from build123d import *
from OCP.BRepAlgoAPI import BRepAlgoAPI_Cut
from OCP.TopTools import TopTools_ListOfShape

# Parameters (mm, degrees)
BOSS_EXTRUDE1_START = -68.064063
BOSS_EXTRUDE1_DEPTH = 898.128125
CUT_EXTRUDE1_START  = -21.828125
SKETCH2_R           = 10.589945851
SKETCH2_R_2         = 7.9375
CUT_EXTRUDE1_DEPTH  = 21.828125
CUT_EXTRUDE2_START  = -898.128125
SKETCH2_2_R         = 10.589945851
SKETCH2_2_R_2       = 7.9375
CUT_EXTRUDE2_DEPTH  = 21.828125


with BuildPart() as part:
    # Sketch1 → Boss-Extrude1 (new body)
    with BuildSketch(Plane.XY.offset(BOSS_EXTRUDE1_START)):
        with BuildLine():
            Line((4.035093565, -9.791065981), (3.586322342, -7.081115612))
            ThreePointArc((3.586322342, -7.081115612), (-1.296798787, 7.830850475), (-1.112187943, -7.859194884))
            Line((-1.112187943, -7.859194884), (-0.663416719, -10.569145253))
            Line((-0.663416719, -10.569145253), (4.035093565, -9.791065981))
        make_face()
    extrude(amount=BOSS_EXTRUDE1_DEPTH)

    # Sketch2 → Cut-Extrude1 (cut)
    with BuildSketch(Plane.XY.offset(830.0640625).offset(CUT_EXTRUDE1_START)):
        Circle(SKETCH2_R)
        with Locations(Location((0, 0, 0), (0, 0, 261.945315936))):
            Circle(SKETCH2_R_2, mode=Mode.SUBTRACT)
    extrude(amount=CUT_EXTRUDE1_DEPTH, mode=Mode.SUBTRACT)


with BuildPart() as cut_extrude2_tool:
    # Sketch2<2> → Cut-Extrude2 (new body)
    with BuildSketch(Plane.XY.offset(830.0640625).offset(CUT_EXTRUDE2_START)):
        Circle(SKETCH2_2_R)
        with Locations(Location((0, 0, 0), (0, 0, 180))):
            Circle(SKETCH2_2_R_2, mode=Mode.SUBTRACT)
    extrude(amount=CUT_EXTRUDE2_DEPTH)


with BuildPart() as part_1:
    add(part.part)

    # Cut-Extrude2: cut by cut_extrude2_tool, with a tolerance
    cut_extrude2_stock = TopTools_ListOfShape()
    cut_extrude2_stock.Append(part_1.part.wrapped)
    cut_extrude2_tools = TopTools_ListOfShape()
    cut_extrude2_tools.Append(cut_extrude2_tool.part.wrapped)
    cut_extrude2_cut = BRepAlgoAPI_Cut()
    cut_extrude2_cut.SetArguments(cut_extrude2_stock)
    cut_extrude2_cut.SetTools(cut_extrude2_tools)
    cut_extrude2_cut.SetFuzzyValue(0.00001)
    cut_extrude2_cut.Build()
    add(Compound.cast(cut_extrude2_cut.Shape()).solids(), mode=Mode.REPLACE)


solid = part_1.part
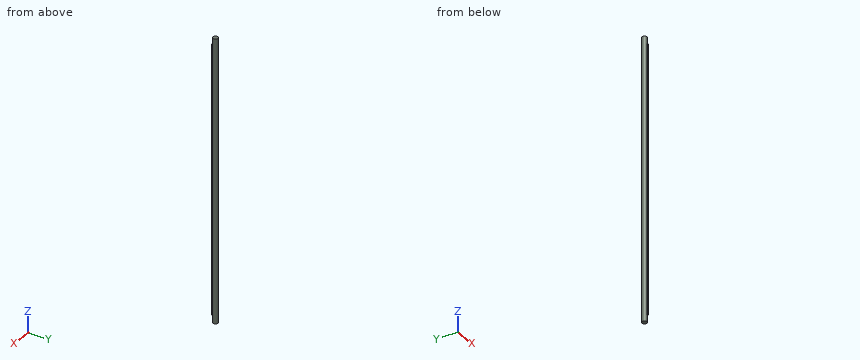
Input: part model. Units: mm. Frame: model coordinates. Round coordinates to 2 decimals unless told otherwise and drop trailing zeros. Loops run counter-clockwise (first coordinate to the right, second up) from the corner with the lowest first, then second, coordinate; pieces in that order, holes last. Notation, with made-up numbers: M 83,39 L 123,39 A17 cw 123,50 Z; hole C -37.5,-6 d9. An arc over 180 degrees is marked long. Answer as CSV lines item,"result". Start each with the question number.
(1) Section B-B, the plane y = 3. Output: boundary loops of the cut face in (x, z).
(2) First-contact query: pin 1 (5 mm diameter, centred on x = 5, z = 469, fed in from -Y); pin 2 (1.5 mm diameter, centred on x = 1, z = 511.5, fed in from -Y); pin 3 (1 mm diameter, centred on x = 1.5, z = 134.5, fed in from +Y). Flat tips, straight axial feed; report the tip coordinate or a pass-through.
(3) Line query: line 1 (X direction, y = -0.5, z = 663); line 2 (Y direction, x = -0.5, z = 501); line 3 (Y direction, x = -5.75, z = 663). Output: solid intervals per line, ascending. Write a range as [from, to].
(4) Section A-A, the plane z = 81. Output: boundary loops of the cut face in (x, y) (1 decimal).
Values found:
1,outline,"M -7.35,-68.06 L 7.35,-68.06 L 7.35,830.06 L -7.35,830.06 Z"
2,pin 1,"stops at y = -10.05"
2,pin 2,"stops at y = -10.42"
2,pin 3,"stops at y = 7.87"
3,line 1,"x = [-7.92, 7.92]"
3,line 2,"y = [-10.54, 7.92]"
3,line 3,"y = [-5.47, 5.47]"
4,outline,"M -1.1,-7.9 L -0.7,-10.6 L 4,-9.8 L 3.6,-7.1 A7.9 ccw long Z"
